For this review, use the dimensioned drawing (mm, ordinates from the lowest corner) and the shaded views. A direction names the side the tool comes from. Coordinates: 2 decimals unless noted, no trailing zeros. Order: outer loops, then holes, each group sorted by start corner. A loop starts at its lowest first (then second) coordinate and runs counter-clockwise, first axis right, second up. Notation, with made-up numbers: (5.25, 45.5) -> (33.25, 45.5) arc R13 cw to (33.25, 51.5) -> close; hole circle Ø2 at (-11, -16.75). An arc over 180 degrees is marked (long way). Use one line per item in the form item = value. Start each with the question number.
(1) Wall thickness on line 1 along X through (y, z) = (40, 125); line 2 along X through (y, z) = (7, 128); line 3 along Z through (x, y) = (128, 30): over which ranges is each line inside the solid? List them lowest first.
(2) For the marked faces 1 and 2, list the 3-axis set-ups (+Z, -Z, +X, -X, +Y, -Y) from which the entire face can be reached by the end or side of a thin tool; tool diameter is ignored.
(3) Take a section at D-D (z = 162). State the section outline as (x, y) points.
(4) Take a section at A-A (z = 128.75). State the section outline as (x, y) points.
(5) Mouldability with a two-part tool opening along X and no side actions: class the marked faces 3, 4 and 5 as +X half, -X half, draft (parallel to the pull), parting line (faces both ways), or undercut.
(6) Take a section at C-C (y = 29). State the section outline as (x, z) points, then the cut area to 3 significant figures.
(7) Take a section at B-B (x = 128.75). State the section outline as (y, z) points.
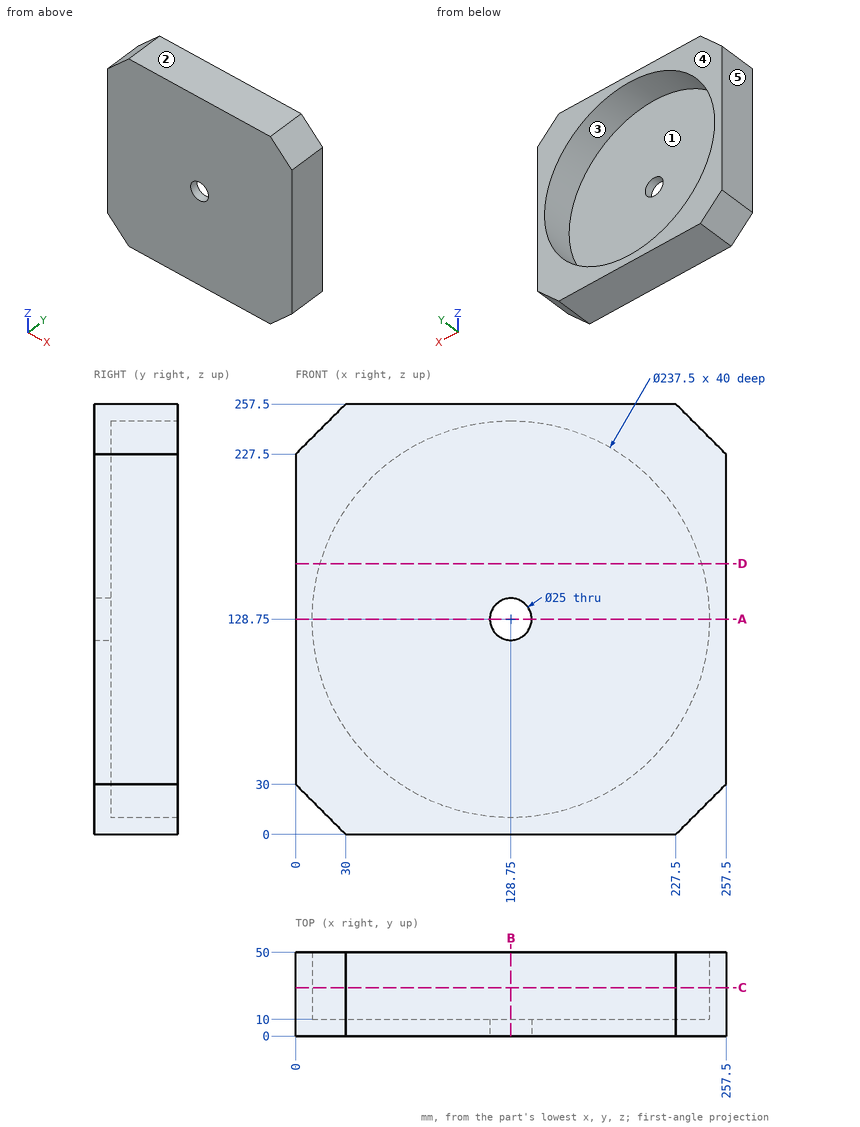
Findings:
q1.line_1 = 0 to 10.06, 247.44 to 257.5
q1.line_2 = 0 to 116.27, 141.23 to 257.5
q1.line_3 = 0 to 10, 247.5 to 257.5
q2.face_1 = +Y
q2.face_2 = +Z, +X, -X, +Y, -Y
q3.outline = (0, 0) -> (257.5, 0) -> (257.5, 50) -> (242.75, 50) -> (242.75, 10) -> (14.75, 10) -> (14.75, 50) -> (0, 50) -> close
q4.outline = (0, 0) -> (116.25, 0) -> (116.25, 10) -> (10, 10) -> (10, 50) -> (0, 50) -> close; (141.25, 0) -> (257.5, 0) -> (257.5, 50) -> (247.5, 50) -> (247.5, 10) -> (141.25, 10) -> close
q5.face_3 = undercut
q5.face_4 = draft
q5.face_5 = -X half
q6.outline = (0, 30) -> (30, 0) -> (227.5, 0) -> (257.5, 30) -> (257.5, 227.5) -> (227.5, 257.5) -> (30, 257.5) -> (0, 227.5) -> close; hole circle Ø237.5 at (128.75, 128.75)
q6.area = 20,200 mm²
q7.outline = (0, 0) -> (50, 0) -> (50, 10) -> (10, 10) -> (10, 116.25) -> (0, 116.25) -> close; (0, 141.25) -> (10, 141.25) -> (10, 247.5) -> (50, 247.5) -> (50, 257.5) -> (0, 257.5) -> close
